Work out the finished part from the listing and answer in its coordinate system (mm). A direction names the side the tool comes from. Give positions to 0.01 mm unless a question says otherwise; leave off trailing zeros. Order: outer loops, then holes, each group sorted by start corner. A loop starts at its lowest first (then second) coordinate and runs counter-clockwise, first axis right, second up. Notation, with made-up numbers: (46, 61) - (92, 61) arc R10 ccw to (92, 69) - close; hole circle Ø5 at (-35.75, 83). An arc over 180 degrees is marked (long way). Write each question's results on one line, items separated by ' | '.
from build123d import *

# Parameters (mm, degrees)
BOSS_EXTRUDE1_DEPTH = 38.1
SKETCH2_R           = 2.0193
CUT_EXTRUDE1_DEPTH  = 38.862
BOSS_EXTRUDE2_DEPTH = 38.1
FILLET1_R           = 3.175
CIRPATTERN1_COUNT   = 2
CIRPATTERN1_ANGLE   = 90
SKETCH6_R           = 1.625
CUT_EXTRUDE2_DEPTH  = 28.575


with BuildPart() as part:
    # Sketch1 → Boss-Extrude1 (new body)
    with BuildSketch(Plane(origin=(0, 0, 0), x_dir=(0, 0, -1), z_dir=(1, 0, 0))):
        Polygon((-12.7, 12.7), (12.7, 12.7), (12.7, -12.7), (-12.7, -12.7), (-12.7, -15.875), (15.875, -15.875), (15.875, 15.875), (-12.7, 15.875), align=None)
    extrude(amount=BOSS_EXTRUDE1_DEPTH)

    # Sketch2 → Cut-Extrude1 (cut)
    with BuildSketch(Plane(origin=(0, 15.875, 0), x_dir=(1, 0, 0), z_dir=(0, 1, 0))):
        with Locations((6.35, 0)):
            Circle(SKETCH2_R)
        with Locations((31.75, 0)):
            Circle(SKETCH2_R)
    cut_extrude1 = extrude(amount=-CUT_EXTRUDE1_DEPTH, mode=Mode.SUBTRACT)

    # Sketch5 → Boss-Extrude2 (add)
    with BuildSketch(Plane(origin=(38.1, 0, 0), x_dir=(0, 0, -1), z_dir=(1, 0, 0))):
        Polygon((15.875, 15.875), (36.45820813, 33.146238), (32.376524054, 38.010634684), (5.996111961, 15.875), align=None)
    extrude(amount=-BOSS_EXTRUDE2_DEPTH)

    # Fillet1
    fillet1_edges = [part.edges().sort_by_distance(p)[0] for p in [
        (19.05, 15.875, -15.875),
        (19.05, 15.875, -5.996111961),
    ]]
    fillet(fillet1_edges, radius=FILLET1_R)

    # CirPattern1: Cut-Extrude1 ×2 about axis
    cirpattern1_axis = Axis((21.2725, 0, 0), (-1, 0, 0))
    for i in range(1, CIRPATTERN1_COUNT):
        add(cut_extrude1.rotate(cirpattern1_axis, i * CIRPATTERN1_ANGLE / (CIRPATTERN1_COUNT - 1)), mode=Mode.SUBTRACT)

    # Sketch6 → Cut-Extrude2 (cut)
    with BuildSketch(Plane(origin=(0, 6.363382753, 5.339473678), x_dir=(1, 0, 0), z_dir=(0, 0.766046722, 0.642784894))):
        with Locations((7.95, 36.134591901)):
            Circle(SKETCH6_R)
        with Locations((30.15, 46.434591901)):
            Circle(SKETCH6_R)
    extrude(amount=-CUT_EXTRUDE2_DEPTH, mode=Mode.SUBTRACT)


solid = part.part
1. A cutting plane is placed at A-A, the plane y = 0. Write down the section's boundary in (x, z) (3 decimals).
Answer list:
outline: (0, -15.875) - (4.331, -15.875) - (4.331, -12.7) - (0, -12.7) - close; (8.369, -15.875) - (29.731, -15.875) - (29.731, -12.7) - (8.369, -12.7) - close; (33.769, -15.875) - (38.1, -15.875) - (38.1, -12.7) - (33.769, -12.7) - close
2. Straight lines are drawn through the part: line 1 (X direction, y = 14.85, z = 0); line 2 (Y direction, x = 28.5, z = -3) (3 decimals); line 3 (Z direction, x = 31.75, y = 13.45) (3 decimals). For each, find the intervals that lie inside material, in ascending order. Write a range as [from, to].
Answer list:
line 1: [0, 4.33], [8.37, 29.73], [33.77, 38.1] | line 2: [-15.875, -12.7], [12.7, 15.875] | line 3: [-15.875, -2.019], [2.019, 12.7]
3. A cutting plane is placed at C-C, the plane z = -8.5. Write down the section's boundary in (x, y) (3 decimals).
Answer list:
outline: (0, -15.875) - (38.1, -15.875) - (38.1, -12.7) - (0, -12.7) - close; (0, 12.7) - (38.1, 12.7) - (38.1, 17.976) - (0, 17.976) - close
4. A cutting plane is placed at D-D, the plane x = 12. Write down the section's boundary in (y, z) (3 decimals).
Answer list:
outline: (-15.875, -15.875) - (14.394, -15.875) arc R3.175 cw to (16.827, -17.009) - (33.146, -36.458) - (38.011, -32.377) - (16.618, -6.881) arc R3.175 cw to (15.875, -4.841) - (15.875, 12.7) - (12.7, 12.7) - (12.7, -12.7) - (-12.7, -12.7) - (-12.7, 12.7) - (-15.875, 12.7) - close
5. A tool of negligible diameter and unlimited length cuts with its end or side. For faces 5 (the face through (19, 0, -12.7)), 6 (the face through (30.9, 32.886, -31.139)), 7 (the face through (19.32, 35.54, -34.45)), 8 (the face through (19, -1, -15.875)), 9 (the face through (19, 15.875, 4)), from which of +Z, -Z, +X, -X, +Y, -Y can it reach the whole face along a straight path? Write none if from no direction.
Answer list:
face 5: +Z, +X, -X | face 6: none | face 7: -Z, +X, -X, +Y | face 8: -Z, +X, -X, -Y | face 9: +Z, +X, -X, +Y
6. Determine the mould class of faces 1 (the face through (33.676, -0.607, -14.31)), 2 (the face through (19, 12.7, 0)), 3 (the face through (19.32, 15.75, -16.18)), 4 (the face through (8.276, 14.31, -0.607)) for opening direction Y: +Y half, -Y half, draft (parallel to the pull), parting line (faces both ways), or undercut.
Answer list:
face 1: undercut | face 2: undercut | face 3: -Y half | face 4: draft
7. Given P1, Ø7.5, axis at x = 21.5, z = -1.5, coming from the +Y side; P2, Ø5.5, axis at x = 31.75, y = 0, coming from the -Z side (3 decimals); P3, Ø12.5, axis at x = 25, y = -2, coming from the +Z side, each flat-ended and moving along its own axis, determine where each tip first touches the part or whether it passes through.
Answer list:
P1: y = 15.9 | P2: z = -15.875 | P3: z = -12.7
8. A cutting plane is placed at B-B, the plane z = 0. Write down the section's boundary in (x, y) (3 decimals), then the cut area to 3 significant figures.
Answer list:
outline: (0, -15.875) - (4.331, -15.875) - (4.331, -12.7) - (0, -12.7) - close; (0, 12.7) - (4.331, 12.7) - (4.331, 15.875) - (0, 15.875) - close; (8.369, -15.875) - (29.731, -15.875) - (29.731, -12.7) - (8.369, -12.7) - close; (8.369, 12.7) - (29.731, 12.7) - (29.731, 15.875) - (8.369, 15.875) - close; (33.769, -15.875) - (38.1, -15.875) - (38.1, -12.7) - (33.769, -12.7) - close; (33.769, 12.7) - (38.1, 12.7) - (38.1, 15.875) - (33.769, 15.875) - close | area: 191 mm^2
